```python
from build123d import *

# Parameters (mm, degrees)
SKETCH1_W                = 10
SKETCH1_H                = 15
BOSS_EXTRUDE1_DEPTH      = 115
SKETCH1_5_W              = 10
SKETCH1_5_H              = 15
CUT_EXTRUDE1_DEPTH       = 15
SKETCH6_W                = 15
SKETCH6_H                = 15
BOSS_EXTRUDE3_DEPTH      = 52.5
BOSS_EXTRUDE3_DEPTH_BACK = 67.5
CUT_EXTRUDE2_REACH       = 52.5
SKETCH7_W                = 33
SKETCH7_H                = 40
CUT_EXTRUDE3_DEPTH       = 15


with BuildPart() as part:
    # Sketch1 → Boss-Extrude1 (new body)
    with BuildSketch(Plane.XY):
        with BuildLine():
            Line((-10, 91.362796982), (-10, 106.362796982))
            ThreePointArc((-10, 106.362796982), (-44.318751046, 85.179188449), (-55.235044142, 46.354499282))
            Line((-55.235044142, 46.354499282), (20, 30.362796982))
            Line((20, 30.362796982), (20, 40.362796982))
            Line((20, 40.362796982), (0, 40.362796982))
            ThreePointArc((0, 40.362796982), (-7.071067812, 43.29172917), (-10, 50.362796982))
            Line((-10, 50.362796982), (-10, 76.362796982))
            Line((-10, 76.362796982), (-20, 76.362796982))
            Line((-20, 76.362796982), (-20, 91.362796982))
            Line((-20, 91.362796982), (-10, 91.362796982))
        make_face()
        with BuildLine():
            Line((20, 30.362796982), (-55.235044142, 46.354499282))
            ThreePointArc((-55.235044142, 46.354499282), (-44.184418834, 18.185611269), (-20, 0))
            Line((-20, 0), (-20, 25.362796982))
            Line((-20, 25.362796982), (20, 25.362796982))
            Line((20, 25.362796982), (20, 30.362796982))
        make_face()
        with Locations((-15, 83.862796982)):
            Rectangle(SKETCH1_W, SKETCH1_H)
    extrude(amount=-BOSS_EXTRUDE1_DEPTH)

    # Sketch1<5> → Cut-Extrude1 (cut)
    with BuildSketch(Plane.XY):
        with BuildLine():
            Line((-10, 91.362796982), (-10, 106.362796982))
            ThreePointArc((-10, 106.362796982), (-44.318751046, 85.179188449), (-55.235044142, 46.354499282))
            Line((-55.235044142, 46.354499282), (20, 30.362796982))
            Line((20, 30.362796982), (20, 40.362796982))
            Line((20, 40.362796982), (0, 40.362796982))
            ThreePointArc((0, 40.362796982), (-7.071067812, 43.29172917), (-10, 50.362796982))
            Line((-10, 50.362796982), (-10, 76.362796982))
            Line((-10, 76.362796982), (-20, 76.362796982))
            Line((-20, 76.362796982), (-20, 91.362796982))
            Line((-20, 91.362796982), (-10, 91.362796982))
        make_face()
        with Locations((-15, 83.862796982)):
            Rectangle(SKETCH1_5_W, SKETCH1_5_H)
    extrude(amount=-CUT_EXTRUDE1_DEPTH, mode=Mode.SUBTRACT)

    # Sketch6 → Boss-Extrude3 (add, two sides)
    with BuildSketch(Plane.XY.offset(-57.5)) as boss_extrude3_sk:
        with Locations((-12.5, 83.862796982)):
            Rectangle(SKETCH6_W, SKETCH6_H)
    extrude(amount=BOSS_EXTRUDE3_DEPTH)
    extrude(boss_extrude3_sk.sketch, amount=-BOSS_EXTRUDE3_DEPTH_BACK)

    # Sketch7 → Cut-Extrude2 (cut, up to next)
    with BuildSketch(Plane(origin=(-5, 0, 0), x_dir=(0, 0, -1), z_dir=(1, 0, 0)), mode=Mode.PRIVATE) as cut_extrude2_sk1:
        with Locations((61.5, 86.362796982)):
            Rectangle(SKETCH7_W, SKETCH7_H)
    cut_extrude2_tool1 = extrude(cut_extrude2_sk1.sketch, amount=-CUT_EXTRUDE2_REACH, mode=Mode.PRIVATE) & part.part
    add(cut_extrude2_tool1.solids().sort_by_distance((-5, 86.362797, -61.5))[0], mode=Mode.SUBTRACT)

    # Sketch8 → Cut-Extrude3 (cut)
    with BuildSketch(Plane(origin=(0, 40.362796982, 0), x_dir=(1, 0, 0), z_dir=(0, 1, 0))):
        with BuildLine():
            Line((5, 25), (5, 105))
            ThreePointArc((5, 105), (10, 110), (15, 105))
            Line((15, 105), (15, 25))
            ThreePointArc((15, 25), (10, 20), (5, 25))
        make_face()
    extrude(amount=-CUT_EXTRUDE3_DEPTH, mode=Mode.SUBTRACT)


solid = part.part
```
Check sheet for the modelled part. Datum: model origin and axes. Units: mm. A direction names the side the tool comes from. Round coordinates to 2 decimals unless told otherwise and drop trailing zeros. Order: outer loops, then holes, each group sorted by start corner. A loop starts at its lowest first (then second) coordinate and runs counter-clockwise, first axis right, second up.
1) Scan lines: line 1 (Z direction, x = -14.5, y = 68); line 2 (Y direction, x = 16.5, z = -108.5); line 3 (Z direction, x = 2, y = 30). Record each from-to range of solid material in increasing order.
2) Mould release check, pull along Z, two halves, no side actions. Record for faces 1 (the flat face through (-26, 28, 0)), 2 (the flat face through (-24, 82, -78)), 3 (the flat face through (-9, 91.363, -106)): +Z half, -Z half, draft (parallel to the pull), parting line (faces both ways), or undercut.
3) Go/stop test with flat-tipped pins: pin 1 Ø2 at (x, z) = (-40, -106) entering from -Y; pin 2 Ø1 at (x, z) = (-10.5, -74) entering from +Y; pin 3 Ø7.5 at (y, z) = (15.5, -50) entering from +X. Record where each tip stops, or that it passes through.
4) Tool access check on faces 4 (the flat face through (-10, 99, -96)), 5 (the flat face through (5, 33, -64)), 6 (the flat face through (-5, 25.363, -57)), 7 (the flat face through (-31, 66.363, -61)). Record the directions out of +Z, -Z, +X, -X, +Y, -Y that give a thin tool (end or side, any length) a straight path to the whole face; none if there is none.
5) Section check B-B (y = 71.5). Record the boundary of the cut face in (x, z), and give its area (3 significant figures).
6) Section check D-D (z = -12). Record the boundary of the cut face in (x, y).
7) Section check A-A (z = -37). Record the boundary of the cut face in (x, y), and give its area (3 significant figures).
8) Section check C-C (x = -37). Record the boundary of the cut face in (y, z), and give its area (3 significant figures).
Result:
1. line 1: z = -115 to -78, -45 to -15
1. line 2: y = 25.36 to 40.36
1. line 3: z = -115 to 0
2. face 1: +Z half
2. face 2: undercut
2. face 3: draft
3. pin 1: stops at y = 12.28
3. pin 2: stops at y = 66.36
3. pin 3: stops at x = -20
4. face 4: +Z, -Z, +X, +Y
4. face 5: +Y, -Y
4. face 6: +Z, -Z, +X, -Y
4. face 7: +X, -X, +Y
5. outline: (-51.88, -115) - (-10, -115) - (-10, -78) - (-51.88, -78) - close; (-51.88, -45) - (-10, -45) - (-10, -15) - (-51.88, -15) - close
5. area: 2,810 mm2
6. outline: (-55.24, 46.35) arc R55.5 ccw to (-20, 0) - (-20, 25.36) - (20, 25.36) - (20, 30.36) - close; (-20, 76.36) - (-5, 76.36) - (-5, 91.36) - (-20, 91.36) - close
7. outline: (-20, 0) - (-20, 25.36) - (5, 25.36) - (5, 40.36) - (0, 40.36) arc R10 cw to (-10, 50.36) - (-10, 76.36) - (-5, 76.36) - (-5, 91.36) - (-10, 91.36) - (-10, 106.36) arc R55.5 ccw to start; (15, 25.36) - (20, 25.36) - (20, 40.36) - (15, 40.36) - close
7. area: 3,860 mm2
8. outline: (10.4, -115) - (93.14, -115) - (93.14, -78) - (66.36, -78) - (66.36, -45) - (93.14, -45) - (93.14, -15) - (42.48, -15) - (42.48, 0) - (10.4, 0) - close
8. area: 7,870 mm2
